Geometry check sheet. Reference: the model listing, model coordinates, mm. Face numbers are marked on the shaded views. A direction names the side the tool comes from. Round coordinates to 2 decimals unless told otherwise and drop trailing zeros. Loops run counter-clockwise (first coordinate to the right, second up) from the corner with the lowest first, then second, coordinate; pieces in that order, holes last. Notation, with made-up numbers: (-32, 20) -> (-11, 20) arc R25 cw to (-11, 45) -> close; hole circle Ø6 at (43, -32). An arc over 180 degrees is marked (long way). Use a Markdown table: item, result. Add a question column.
Q1. Release check for a two-part mould opening along Y. For the marked faces 3, 4 and 5 record: released by +Y, released by -Y, zero draft, split by the parting line, or undercut.
Q2. Sectioned sample at B-B, the plane y = 30. Enter the section's corners in (x, z).
Q3. Material ranges on L1, parallel to X at y = 3, z = 15; L2, parallel to X at y = 10, z = 3.5; L3, parallel to Y at x = 60, z = 7.1 (3 decimals), recorded low to high.
Q4. Sectioned sample at C-C, the plane x = 23.5. Enter the section's corners in (y, z) (3 decimals).
Q5. Gauge pin test, flat ends, axial feed: P1, Ø1, axis at x = 67, y = 27, coming from the +Z side; P2, Ø6, axis at x = 85, y = 30, coming from the +Z side; P3, Ø1.5, axis at x = 2.5, y = 3, coming from the -Z side. Record the tip position at first contact, or that the pin passes through.
Q6. Sectioned sample at A-A, the plane z = 15. Enter the section's corners in (x, y), then the cut area to 3 significant figures.
Q7. Set-up check for the marked faces 1 and 2: record each of +Z, -Z, +X, -X, +Y, -Y from which the full face is reachable in a straight line by a thin tool's end or side.
Q8. Sectioned sample at D-D, the plane z = 29. Enter the section's corners in (x, y).
```python
from build123d import *

# Parameters (mm, degrees)
BOSS_EXTRUDE1_DEPTH     = 10
SKETCH2_R               = 2.6
CUT_EXTRUDE1_DEPTH      = 142.774468788
SKETCH3_W               = 60
SKETCH3_H               = 9
SKETCH3_W_2             = 9
SKETCH3_H_2             = 60
BOSS_EXTRUDE3_DEPTH     = 1.46
CUT_EXTRUDE2_DEPTH      = 142.774468788
CUT_EXTRUDE2_DEPTH_BACK = 142.774468788
SKETCH2_2_R             = 2.6
CHAMFER1_SIZE           = 1.46
CUT_EXTRUDE3_START      = 10
SKETCH4_R               = 4.5
CUT_EXTRUDE3_DEPTH      = 5
SKETCH5_W               = 100
SKETCH5_H               = 50
SKETCH5_R               = 11.5
SKETCH5_R_2             = 1.75
BOSS_EXTRUDE4_DEPTH     = 5
BOSS_EXTRUDE5_DEPTH     = 10
BOSS_EXTRUDE6_START     = 100
BOSS_EXTRUDE6_DEPTH     = 10
CUT_EXTRUDE4_DEPTH      = 154.622914957
CUT_EXTRUDE4_DEPTH_BACK = 154.622914957
SKETCH9_R               = 1.75
SKETCH10_W              = 10
SKETCH10_H              = 5
CUT_EXTRUDE5_DEPTH      = 5
CUT_EXTRUDE6_START      = 100
SKETCH10_2_W            = 10
SKETCH10_2_H            = 5
CUT_EXTRUDE6_DEPTH      = 5
CUT_EXTRUDE7_START      = 60
SKETCH11_W              = 10
SKETCH11_H              = 5
CUT_EXTRUDE7_DEPTH      = 5
CUT_EXTRUDE9_START      = 100
SKETCH12_R              = 3
CUT_EXTRUDE9_DEPTH      = 95
CHAMFER2_SIZE           = 5


# Some blends are built 0.0001 mm under size
with BuildPart() as part:
    # Sketch1 → Boss-Extrude1 (new body)
    with BuildSketch(Plane.XY):
        Polygon((0, 0), (100, 0), (100, 40), (20, 100), (0, 100), align=None)
    extrude(amount=BOSS_EXTRUDE1_DEPTH)

    # Sketch2 → Cut-Extrude1 (cut, through all)
    with BuildSketch(Plane.XY):
        with Locations((10, 85)):
            Circle(SKETCH2_R)
        with Locations((10, 60)):
            Circle(SKETCH2_R)
        with Locations((85, 30)):
            Circle(SKETCH2_R)
        with Locations((85, 10)):
            Circle(SKETCH2_R)
        with Locations((60, 10)):
            Circle(SKETCH2_R)
        with Locations((60, 30)):
            Circle(SKETCH2_R)
    extrude(amount=CUT_EXTRUDE1_DEPTH, mode=Mode.SUBTRACT)

    # Sketch3 → Boss-Extrude3 (add)
    with BuildSketch(Plane.XY):
        with Locations((70, 30)):
            Rectangle(SKETCH3_W, SKETCH3_H)
        with Locations((70, 10)):
            Rectangle(SKETCH3_W, SKETCH3_H)
        with Locations((10, 70)):
            Rectangle(SKETCH3_W_2, SKETCH3_H_2)
    extrude(amount=-BOSS_EXTRUDE3_DEPTH)

    # Sketch2<2> → Cut-Extrude2 (cut, two sides: drawn at the far end of the back side and taken through both)
    with BuildSketch(Plane.XY.offset(-CUT_EXTRUDE2_DEPTH_BACK)):
        with Locations((10, 85)):
            Circle(SKETCH2_2_R)
        with Locations((10, 60)):
            Circle(SKETCH2_2_R)
        with Locations((85, 30)):
            Circle(SKETCH2_2_R)
        with Locations((85, 10)):
            Circle(SKETCH2_2_R)
        with Locations((60, 10)):
            Circle(SKETCH2_2_R)
        with Locations((60, 30)):
            Circle(SKETCH2_2_R)
    extrude(amount=CUT_EXTRUDE2_DEPTH + CUT_EXTRUDE2_DEPTH_BACK, mode=Mode.SUBTRACT)

    # Chamfer1
    chamfer1_edges = [part.edges().sort_by_distance(p)[0] for p in [
        (14.5, 70, -1.46),
        (5.5, 70, -1.46),
        (70, 5.5, -1.46),
        (70, 14.5, -1.46),
        (70, 25.5, -1.46),
        (70, 34.5, -1.46),
    ]]
    chamfer(chamfer1_edges, length=CHAMFER1_SIZE - 0.0001)  # a hair under: the kernel refuses the full size

    # Sketch4 → Cut-Extrude3 (cut)
    with BuildSketch(Plane.XY.offset(CUT_EXTRUDE3_START)):
        with Locations((10, 85)):
            Circle(SKETCH4_R)
        with Locations((10, 60)):
            Circle(SKETCH4_R)
        with Locations((60, 30)):
            Circle(SKETCH4_R)
        with Locations((85, 30)):
            Circle(SKETCH4_R)
        with Locations((85, 10)):
            Circle(SKETCH4_R)
        with Locations((60, 10)):
            Circle(SKETCH4_R)
    extrude(amount=-CUT_EXTRUDE3_DEPTH, mode=Mode.SUBTRACT)

    # Sketch5 → Boss-Extrude4 (add)
    with BuildSketch(Plane(origin=(0, 0, 0), x_dir=(1, 0, 0), z_dir=(0, 1, 0))):
        with Locations((50, -35)):
            Rectangle(SKETCH5_W, SKETCH5_H)
        with Locations(Location((50, -35, 0), (0, 0, 270))):
            Circle(SKETCH5_R, mode=Mode.SUBTRACT)
        with Locations(Location((65.5, -50.5, 0), (0, 0, 270))):
            Circle(SKETCH5_R_2, mode=Mode.SUBTRACT)
        with Locations(Location((34.5, -50.5, 0), (0, 0, 270))):
            Circle(SKETCH5_R_2, mode=Mode.SUBTRACT)
        with Locations(Location((34.5, -19.5, 0), (0, 0, 270))):
            Circle(SKETCH5_R_2, mode=Mode.SUBTRACT)
        with Locations(Location((65.5, -19.5, 0), (0, 0, 270))):
            Circle(SKETCH5_R_2, mode=Mode.SUBTRACT)
    extrude(amount=BOSS_EXTRUDE4_DEPTH)

    # Sketch8 → Boss-Extrude5 (add)
    with BuildSketch(Plane(origin=(0, 0, 0), x_dir=(0, 0, -1), z_dir=(1, 0, 0))):
        Polygon((-10, 5), (-60, 5), (-10, 40), align=None)
    extrude(amount=BOSS_EXTRUDE5_DEPTH)

    # Sketch8<2> → Boss-Extrude6 (add)
    with BuildSketch(Plane(origin=(0, 0, 0), x_dir=(0, 0, -1), z_dir=(1, 0, 0)).offset(BOSS_EXTRUDE6_START)):
        Polygon((-10, 5), (-60, 5), (-10, 40), align=None)
    extrude(amount=-BOSS_EXTRUDE6_DEPTH)

    # Sketch9 → Cut-Extrude4 (cut, two sides: drawn at the far end of the back side and taken through both)
    with BuildSketch(Plane(origin=(0, 0, 0), x_dir=(1, 0, 0), z_dir=(0, 1, 0)).offset(-CUT_EXTRUDE4_DEPTH_BACK)):
        with Locations(Location((5, -55, 0), (0, 0, 270))):
            Circle(SKETCH9_R)
        with Locations(Location((95, -55, 0), (0, 0, 270))):
            Circle(SKETCH9_R)
        with Locations(Location((95, -15, 0), (0, 0, 270))):
            Circle(SKETCH9_R)
        with Locations(Location((5, -15, 0), (0, 0, 270))):
            Circle(SKETCH9_R)
    extrude(amount=CUT_EXTRUDE4_DEPTH + CUT_EXTRUDE4_DEPTH_BACK, mode=Mode.SUBTRACT)

    # Sketch10 → Cut-Extrude5 (cut)
    with BuildSketch(Plane(origin=(0, 0, 0), x_dir=(0, 0, -1), z_dir=(1, 0, 0))):
        with Locations((-30, 2.5)):
            Rectangle(SKETCH10_W, SKETCH10_H)
    extrude(amount=CUT_EXTRUDE5_DEPTH, mode=Mode.SUBTRACT)

    # Sketch10<2> → Cut-Extrude6 (cut)
    with BuildSketch(Plane(origin=(0, 0, 0), x_dir=(0, 0, -1), z_dir=(1, 0, 0)).offset(CUT_EXTRUDE6_START)):
        with Locations((-30, 2.5)):
            Rectangle(SKETCH10_2_W, SKETCH10_2_H)
    extrude(amount=-CUT_EXTRUDE6_DEPTH, mode=Mode.SUBTRACT)

    # Sketch11 → Cut-Extrude7 (cut)
    with BuildSketch(Plane.XY.offset(CUT_EXTRUDE7_START)):
        with Locations((50, 2.5)):
            Rectangle(SKETCH11_W, SKETCH11_H)
    extrude(amount=-CUT_EXTRUDE7_DEPTH, mode=Mode.SUBTRACT)

    # Sketch12 → Cut-Extrude9 (cut)
    with BuildSketch(Plane(origin=(0, 0, 0), x_dir=(1, 0, 0), z_dir=(0, 1, 0)).offset(CUT_EXTRUDE9_START)):
        with Locations((5, -15)):
            Circle(SKETCH12_R)
        with Locations((5, -55)):
            Circle(SKETCH12_R)
        with Locations((95, -55)):
            Circle(SKETCH12_R)
        with Locations((95, -15)):
            Circle(SKETCH12_R)
    extrude(amount=-CUT_EXTRUDE9_DEPTH, mode=Mode.SUBTRACT)

    # Chamfer2
    # the kernel refuses this chamfer: 5 mm, written as the material it takes off along each edge
    with BuildSketch(Plane(origin=(3.333333333, 96.666666667, 6.666666667), x_dir=(-0.7071067811865474, 0, -0.7071067811865476), z_dir=(-0.5773502691896258, 0.5773502691896257, 0.5773502691896257))) as chamfer2_piece_1:
        Polygon((-3.535533906, 2.041241452), (3.535533906, 2.041241452), (0, -4.082482905), align=None)
    extrude(amount=6.350852961, mode=Mode.SUBTRACT)
    with BuildSketch(Plane(origin=(110.286731952, 32.284951036, 10), x_dir=(0.016497525966350957, 0.021996701288467948, -0.9996219169112968), z_dir=(-0.8000000000000002, 0.6, 0))) as chamfer2_piece_2_section:
        Polygon((CHAMFER2_SIZE * 0.999621916911, CHAMFER2_SIZE * 0.0274958766106), (-CHAMFER2_SIZE * 0.0274958766106, CHAMFER2_SIZE * 0.999621916911), (0, 0), align=None)
    chamfer2_piece_2 = extrude(amount=125.71682988, mode=Mode.PRIVATE)
    chamfer2_piece_2 = split(chamfer2_piece_2, bisect_by=Plane(origin=(56.438385269, 50.830938552, -5.472769359), z_dir=(0, 0.8192319205190406, 0.5734623443633283)), keep=Keep.TOP, mode=Mode.PRIVATE)
    add(chamfer2_piece_2, mode=Mode.SUBTRACT)
    with BuildSketch(Plane(origin=(100, -12.85841494, 60), x_dir=(0.0274958766105877, 0, -0.9996219169112968), z_dir=(0, 1, 0))) as chamfer2_piece_3:
        Polygon((CHAMFER2_SIZE * 0.999621916911, CHAMFER2_SIZE * 0.0274958766106), (-CHAMFER2_SIZE * 0.0274958766106, CHAMFER2_SIZE * 0.999621916911), (0, 0), align=None)
    extrude(amount=30.71682988, mode=Mode.SUBTRACT)
    with BuildSketch(Plane(origin=(0, -12.85841494, 60), x_dir=(-0.027495876610586372, 0, -0.9996219169112968), z_dir=(0, 1, 0))) as chamfer2_piece_4:
        Polygon((CHAMFER2_SIZE * 0.999621916911, -CHAMFER2_SIZE * 0.0274958766106), (-CHAMFER2_SIZE * 0.0274958766106, -CHAMFER2_SIZE * 0.999621916911), (0, 0), align=None)
    extrude(amount=30.71682988, mode=Mode.SUBTRACT)
    with BuildSketch(Plane(origin=(32.85841494, 100, 10), x_dir=(0, 0.0274958766105877, -0.9996219169112968), z_dir=(-1, 0, 0))) as chamfer2_piece_5:
        Polygon((CHAMFER2_SIZE * 0.999621916911, CHAMFER2_SIZE * 0.0274958766106), (-CHAMFER2_SIZE * 0.0274958766106, CHAMFER2_SIZE * 0.999621916911), (0, 0), align=None)
    extrude(amount=45.71682988, mode=Mode.SUBTRACT)
    with BuildSketch(Plane(origin=(0, 112.85841494, 10), x_dir=(-0.02749587661058638, 0, -0.9996219169112968), z_dir=(0, -1, 0))) as chamfer2_piece_6_section:
        Polygon((CHAMFER2_SIZE * 0.999621916911, CHAMFER2_SIZE * 0.0274958766106), (-CHAMFER2_SIZE * 0.0274958766106, CHAMFER2_SIZE * 0.999621916911), (0, 0), align=None)
    chamfer2_piece_6 = extrude(amount=85.71682988, mode=Mode.PRIVATE)
    chamfer2_piece_6 = split(chamfer2_piece_6, bisect_by=Plane(origin=(1.674929178, 50.830938552, -5.472769359), z_dir=(0, 0.8192319205190406, 0.5734623443633283)), keep=Keep.TOP, mode=Mode.PRIVATE)
    add(chamfer2_piece_6, mode=Mode.SUBTRACT)
    with BuildSketch(Plane(origin=(0, 100, -12.85841494), x_dir=(-0.027495876610586313, -0.9996219169112968, 0), z_dir=(0, 0, 1))) as chamfer2_piece_7:
        Polygon((CHAMFER2_SIZE * 0.999621916911, CHAMFER2_SIZE * 0.0274958766106), (-CHAMFER2_SIZE * 0.0274958766106, CHAMFER2_SIZE * 0.999621916911), (0, 0), align=None)
    extrude(amount=35.71682988, mode=Mode.SUBTRACT)


solid = part.part
```
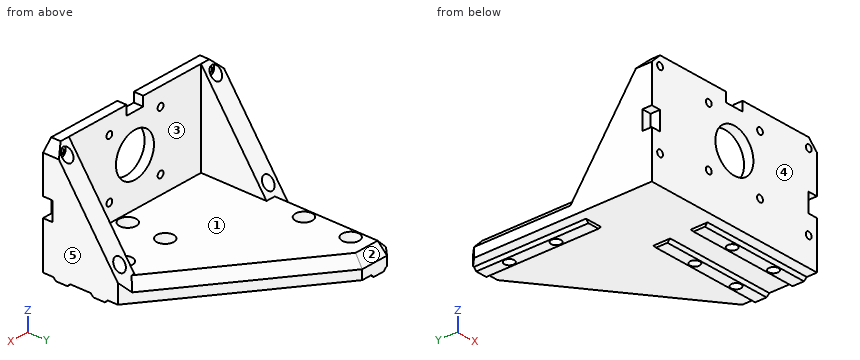
Values:
| question | item | result |
|---|---|---|
| 1 | face 3 | released by +Y |
| 1 | face 4 | released by -Y |
| 1 | face 5 | zero draft |
| 2 | outline | (0, 0) -> (40, 0) -> (40, -1.46) -> (57.4, -1.46) -> (57.4, 5) -> (55.5, 5) -> (55.5, 10) -> (10, 10) -> (10, 24.29) -> (0, 24.29) -> close; (62.6, -1.46) -> (82.4, -1.46) -> (82.4, 5) -> (80.5, 5) -> (80.5, 10) -> (64.5, 10) -> (64.5, 5) -> (62.6, 5) -> close; (87.6, -1.46) -> (100, -1.46) -> (100, 24.29) -> (90, 24.29) -> (90, 10) -> (89.5, 10) -> (89.5, 5) -> (87.6, 5) -> close; hole circle Ø6 at (5, 15); hole circle Ø6 at (95, 15) |
| 3 | L1 | 0 to 3.25, 6.75 to 93.25, 96.75 to 100 |
| 3 | L2 | 0 to 57.4, 62.6 to 82.4, 87.6 to 100 |
| 3 | L3 | 0 to 5.5, 14.5 to 25.5, 34.5 to 67.375 |
| 4 | outline | (0, 0) -> (97.375, 0) -> (97.375, 5) -> (91.125, 10) -> (5, 10) -> (5, 60) -> (0, 60) -> close |
| 5 | P1 | z = 10 |
| 5 | P2 | z = 5 |
| 5 | P3 | z = 0 |
| 6 | outline | (0, 0) -> (3.25, 0) -> (3.25, 5) -> (2, 5) -> (2, 36.5) -> (0, 36.5) -> close; (6.75, 0) -> (93.25, 0) -> (93.25, 5) -> (92, 5) -> (92, 36.5) -> (90, 36.5) -> (90, 5) -> (10, 5) -> (10, 36.5) -> (8, 36.5) -> (8, 5) -> (6.75, 5) -> close; (96.75, 0) -> (100, 0) -> (100, 36.5) -> (98, 36.5) -> (98, 5) -> (96.75, 5) -> close |
| 6 | area | 717 mm^2 |
| 7 | face 1 | +Z, +Y |
| 7 | face 2 | +Z, +X, -X, +Y |
| 8 | outline | (0, 5) -> (5, 5) -> (5, 0) -> (40.19, 0) -> (40.19, 5) -> (10, 5) -> (10, 26.7) -> (0, 26.7) -> close; (59.81, 0) -> (95, 0) -> (95, 5) -> (100, 5) -> (100, 26.7) -> (90, 26.7) -> (90, 5) -> (59.81, 5) -> close |
